Geometry: final body of the model. Coordinates: model frame, mm. Round coordinates to 2 decimals unless told otherwise and drop trailing zeros. Loops run counter-clockwise (first coordinate to the right, second up) from the corner with the lowest first, then second, coordinate; pieces in that order, holes last. Notation, with made-up numbers: (89, -10.5) -> (123, -10.5) arc R29 ccw to (123, 24.5) -> close; hole circle Ø10 at (14, 21). An arc over 180 degrees is marked (long way). Answer in a Markdown table with one row per item.
```python
from build123d import *

# Parameters (mm, degrees)
SKETCH1_W            = 20.4978
SKETCH1_H            = 45.599133257
SKETCH1_R            = 0.890894817
SKETCH1_R_2          = 0.963661062
BOSS_EXTRUDE1_DEPTH  = 3.175
M5_CLEARANCE_HOLE3_D = 5.8
FILLET1_R            = 2.54
M5_CLEARANCE_HOLE1_D = 5.8


with BuildPart() as part:
    # Sketch1 → Boss-Extrude1 (new body)
    with BuildSketch(Plane.XY):
        with Locations((19.037900458, -1.288082074)):
            Rectangle(SKETCH1_W, SKETCH1_H)
        with Locations((19.037900458, -11.349548702)):
            Circle(SKETCH1_R, mode=Mode.SUBTRACT)
        with Locations((19.037900458, 11.262584555)):
            Circle(SKETCH1_R_2, mode=Mode.SUBTRACT)
    extrude(amount=BOSS_EXTRUDE1_DEPTH)

    # M5 Clearance Hole3 (through all)
    with Locations(Plane.XY.offset(3.175)):
        with Locations((19.037900458, 11.262584555)):
            Hole(M5_CLEARANCE_HOLE3_D / 2)

    # Fillet1
    fillet1_edges = [part.edges().sort_by_distance(p)[0] for p in [
        (29.286800458, 21.511484555, 1.5875),
        (29.286800458, -24.087648702, 1.5875),
        (8.789000458, -24.087648702, 1.5875),
        (8.789000458, 21.511484555, 1.5875),
    ]]
    fillet(fillet1_edges, radius=FILLET1_R)

    # M5 Clearance Hole1 (through all)
    with Locations(Plane.XY.offset(3.175)):
        with Locations((19.037900458, -11.349548702)):
            Hole(M5_CLEARANCE_HOLE1_D / 2)


solid = part.part
```
Item 1: Draft query along Y for faces 1 (the face through (19, -1, 0)), 2 (the face through (17.48, 13.71, 1.57)), 3 (the face through (9.51, -23.32, 1.61)), 4 (the face through (17.479, -8.904, 1.565)). Return one class per face: pulls with the +Y half, pulls with the -Y half, needs draft (parallel to the pull), parting line crosses it, or undercut.
Answer:
| item | result |
|---|---|
| face 1 | needs draft |
| face 2 | undercut |
| face 3 | pulls with the -Y half |
| face 4 | undercut |
Item 2: Cut plane A-A (x = 20.75). Output: boundary loops of the cut face in (y, z) (3 decimals).
Answer:
| item | result |
|---|---|
| outline | (-24.088, 0) -> (-13.69, 0) -> (-13.69, 3.175) -> (-24.088, 3.175) -> close; (-9.009, 0) -> (8.922, 0) -> (8.922, 3.175) -> (-9.009, 3.175) -> close; (13.603, 0) -> (21.511, 0) -> (21.511, 3.175) -> (13.603, 3.175) -> close |
Item 3: Cut plane B-B (z = 2.1). Output: boundary loops of the cut face in (x, y).
Answer:
| item | result |
|---|---|
| outline | (8.79, -21.55) arc R2.54 ccw to (11.33, -24.09) -> (26.75, -24.09) arc R2.54 ccw to (29.29, -21.55) -> (29.29, 18.97) arc R2.54 ccw to (26.75, 21.51) -> (11.33, 21.51) arc R2.54 ccw to (8.79, 18.97) -> close; hole circle Ø5.8 at (19.04, -11.35); hole circle Ø5.8 at (19.04, 11.26) |
Item 4: Pin query (flat end, axial travel): pin 1 Ø1 at (x, y) = (23.5, -3) entering from -Z. Return the tip coordinate at first contact, or that it passes through.
Answer:
| item | result |
|---|---|
| pin 1 | stops at z = 0 |
Item 5: Line query: probe 1 along Y at (x, z) = (20.25, 1.1) (3 decimals); probe 2 along X at (y, z) = (12, 1.35); probe 3 along X at (y, z) = (12.5, 0.7). Output: solid intervals per line, ascending. Write a range as [from, to].
Answer:
| item | result |
|---|---|
| probe 1 | y = [-24.088, -13.984], [-8.715, 8.628], [13.897, 21.511] |
| probe 2 | x = [8.79, 16.23], [21.84, 29.29] |
| probe 3 | x = [8.79, 16.42], [21.66, 29.29] |
